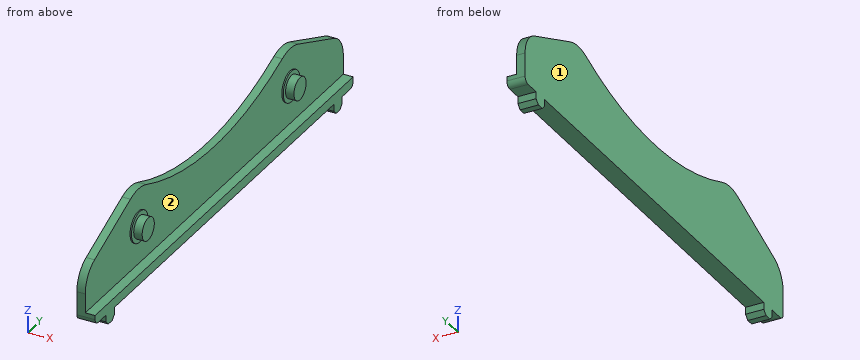
```python
from build123d import *

# Parameters (mm, degrees)
F1_DEPTH = 3
F2_W     = 170
F2_H     = 3.5
F2_R     = 4
F3_DEPTH = 3.5
F4_R     = 5.5
F4_R_2   = 4
F5_DEPTH = 0.5
F6_R     = 2


with BuildPart() as f1:
    # F0 (on Right) → F1 (new body)
    with BuildSketch(Plane.YZ):
        with BuildLine():
            ThreePointArc((-78.857143, 19.568113), (-83.323804, 15.883977), (-85, 10.34193))
            Line((-85, 10.34193), (-85, 0))
            Line((-85, 0), (-77.75, 0))
            Line((-77.75, 0), (-72.25, 0))
            Line((-72.25, 0), (72.25, 0))
            Line((72.25, 0), (77.75, 0))
            Line((77.75, 0), (85, 0))
            Line((85, 0), (85, 10.34193))
            ThreePointArc((85, 10.34193), (83.323804, 15.883977), (78.857143, 19.568113))
            Line((78.857143, 19.568113), (55.207143, 29.455347))
            ThreePointArc((55.207143, 29.455347), (50, 30.5), (44.792857, 29.455347))
            ThreePointArc((44.792857, 29.455347), (0, 20.469036), (-44.792857, 29.455347))
            ThreePointArc((-44.792857, 29.455347), (-50, 30.5), (-55.207143, 29.455347))
            Line((-55.207143, 29.455347), (-78.857143, 19.568113))
        make_face()
        Polygon((-72.25, 0), (-77.75, 0), (-77.75, -2.5), (-76.25, -4), (-73.75, -4), (-72.25, -2.5), align=None)
        Polygon((77.75, 0), (72.25, 0), (72.25, -2.5), (73.75, -4), (76.25, -4), (77.75, -2.5), align=None)
    extrude(amount=-F1_DEPTH)

    # F2 (on face) + F0 (on Right) → F3 (join)
    with BuildSketch(Plane.YZ):
        with Locations((0, 1.75)):
            Rectangle(F2_W, F2_H)
        with Locations((-50, 17)):
            Circle(F2_R)
        with Locations((50, 17)):
            Circle(F2_R)
    with BuildSketch(Plane.YZ):
        Polygon((-72.25, 0), (-77.75, 0), (-77.75, -2.5), (-76.25, -4), (-73.75, -4), (-72.25, -2.5), align=None)
        Polygon((77.75, 0), (72.25, 0), (72.25, -2.5), (73.75, -4), (76.25, -4), (77.75, -2.5), align=None)
    extrude(amount=F3_DEPTH)

    # F4 (on Right) → F5 (join)
    with BuildSketch(Plane.YZ):
        with Locations((-50, 17)):
            Circle(F4_R)
        with Locations((-50, 17)):
            Circle(F4_R_2, mode=Mode.SUBTRACT)
        with Locations((50, 17)):
            Circle(F4_R)
        with Locations((50, 17)):
            Circle(F4_R_2, mode=Mode.SUBTRACT)
    extrude(amount=F5_DEPTH)

    # F6
    f6_edges = [f1.edges().sort_by_distance(p)[0] for p in [
        (0.25, -85, 0),
        (0.25, 85, 0),
    ]]
    fillet(f6_edges, radius=F6_R)


solid = f1.part
```
Work out the finished part from the listing and answer in its coordinate system (mm). Face numbers are marked on the shaded views. Coordinates: 2 decimals unless noted, no trailing zeros. Order: outer loops, then holes, each group sorted by start corner. A loop starts at its lowest first (then second) coordinate and runs counter-clockwise, first axis right, second up. Notation, with made-up numbers: (84, 83.5) - (130, 83.5) arc R36 ccw to (130, 122.5) - close; hole circle Ø2 at (60, 71.25). An arc over 180 degrees is marked (long way). Answer as a JSON object with one key per item and string values.
1. Find section C-C on z = 17. Determine the outline of the cut face in (x, y), plus the area to 3 significant figures.
Output values:
{"outline": "(-3, -82.46) - (0, -82.46) - (0, -55.5) - (0.5, -55.5) - (0.5, -54) - (3.5, -54) - (3.5, -46) - (0.5, -46) - (0.5, -44.5) - (0, -44.5) - (0, 44.5) - (0.5, 44.5) - (0.5, 46) - (3.5, 46) - (3.5, 54) - (0.5, 54) - (0.5, 55.5) - (0, 55.5) - (0, 82.46) - (-3, 82.46) - close", "area": "554 mm²"}
2. Each of these flat-tipped pins is pushed along its axis until it touches: P1, Ø1.2, axis at x = 1.5, z = -1.5, coming from the +Y side; P2, Ø1.2, axis at x = 2, z = -1.5, coming from the -Y side; P3, Ø1.5, axis at x = 1.5, y = -53.5, coming from the +Z side. Where does it stop, or does it pass through?
Output values:
{"P1": "stops at y = 77.75", "P2": "stops at y = -77.75", "P3": "stops at z = 19.9"}
3. Find section B-B on y = -50. Determine the outline of the cut face in (x, z), plus the area to 3 significant figures.
Output values:
{"outline": "(-3, 0) - (3.5, 0) - (3.5, 3.5) - (0, 3.5) - (0, 11.5) - (0.5, 11.5) - (0.5, 13) - (3.5, 13) - (3.5, 21) - (0.5, 21) - (0.5, 22.5) - (0, 22.5) - (0, 30.5) - (-3, 30.5) - close", "area": "133 mm²"}
4. Consider line 1 (Z direction, x = 1.5, y = -71.5); line 2 (X direction, y = 26.5, z = 12.5); line 3 (Z direction, x = -2.25, y = -49.5). Determine where each line is inside the solid, lowest interval first.
Output values:
{"line 1": "z = 0 to 3.5", "line 2": "x = -3 to 0", "line 3": "z = 0 to 30.49"}
5. The mould has two halves that part along Y. Classify the marked faces 1 and 2: +Y half, -Y half, draft (parallel to the pull), parting line (faces both ways), or undercut.
Output values:
{"face 1": "draft", "face 2": "undercut"}
6. Find section D-D on y = -2. Determine the outline of the cut face in (x, z).
Output values:
{"outline": "(-3, 0) - (3.5, 0) - (3.5, 3.5) - (0, 3.5) - (0, 20.49) - (-3, 20.49) - close"}
7. Find section A-A on x = 1.5. Determine the outline of the cut face in (y, z), plus the area to 3 significant figures.
Output values:
{"outline": "(-85, 2) arc R2 ccw to (-83, 0) - (-77.75, 0) - (-77.75, -2.5) - (-76.25, -4) - (-73.75, -4) - (-72.25, -2.5) - (-72.25, 0) - (72.25, 0) - (72.25, -2.5) - (73.75, -4) - (76.25, -4) - (77.75, -2.5) - (77.75, 0) - (83, 0) arc R2 ccw to (85, 2) - (85, 3.5) - (-85, 3.5) - close; circle Ø8 at (-50, 17); circle Ø8 at (50, 17)", "area": "733 mm²"}
